Source: CAD feature listing. Evaluate the final solid. Frame: model axes, mm. A direction names the side the tool comes from. Give positions to 0.01 mm unless a question says otherwise; leave off trailing zeros. Order: outer loops, then holes, each group sorted by start corner. A loop starts at its lowest first (then second) coordinate and runs counter-clockwise, first axis right, second up.
from build123d import *

# Parameters (mm, degrees)
SKETCH_W        = 108
SKETCH_H        = 38
PAD_DEPTH       = 3
SKETCH002_W     = 3
SKETCH002_H     = 38
POCKET_DEPTH    = 1.5
SKETCH003_W     = 3
SKETCH003_H     = 38
POCKET001_DEPTH = 1.5
SKETCH004_W     = 102
SKETCH004_H     = 1.5
POCKET002_DEPTH = 1.5
SKETCH005_W     = 102
SKETCH005_H     = 1.5
POCKET003_DEPTH = 1.5
SKETCH006_W     = 5
SKETCH006_H     = 5
POCKET004_DEPTH = 3


with BuildPart() as part:
    # Sketch → Pad (new body)
    with BuildSketch(Plane.XY):
        with Locations((54, -19)):
            Rectangle(SKETCH_W, SKETCH_H)
    extrude(amount=PAD_DEPTH)

    # Sketch002 (on Face6 of Pad) → Pocket (cut)
    with BuildSketch(Plane.XY.offset(3)):
        with Locations((1.5, -19)):
            Rectangle(SKETCH002_W, SKETCH002_H)
    extrude(amount=-POCKET_DEPTH, mode=Mode.SUBTRACT)

    # Sketch003 (on Face4 of Pocket) → Pocket001 (cut)
    with BuildSketch(Plane.XY.offset(3)):
        with Locations((106.5, -19)):
            Rectangle(SKETCH003_W, SKETCH003_H)
    extrude(amount=-POCKET001_DEPTH, mode=Mode.SUBTRACT)

    # Sketch004 (on Face6 of Pocket001) → Pocket002 (cut)
    with BuildSketch(Plane.XY.offset(3)):
        with Locations((54, -0.75)):
            Rectangle(SKETCH004_W, SKETCH004_H)
    extrude(amount=-POCKET002_DEPTH, mode=Mode.SUBTRACT)

    # Sketch005 (on Face12 of Pocket002) → Pocket003 (cut)
    with BuildSketch(Plane.XY.offset(3)):
        with Locations((54, -37.25)):
            Rectangle(SKETCH005_W, SKETCH005_H)
    extrude(amount=-POCKET003_DEPTH, mode=Mode.SUBTRACT)

    # Sketch006 (on Face13 of Pocket003) → Pocket004 (cut)
    with BuildSketch(Plane.XY.offset(3)):
        with Locations((6.75, -16.25)):
            Rectangle(SKETCH006_W, SKETCH006_H)
    extrude(amount=-POCKET004_DEPTH, mode=Mode.SUBTRACT)


solid = part.part
1) Section query A-A on y = -17. Output: boundary loops of the cut face in (x, z), and give its area (3 significant figures).
Checks:
outline: (0, 0) - (4.25, 0) - (4.25, 3) - (3, 3) - (3, 1.5) - (0, 1.5) - close; (9.25, 0) - (108, 0) - (108, 1.5) - (105, 1.5) - (105, 3) - (9.25, 3) - close
area: 300 mm2
2) Ray query, L1, parallel to X at y = -22.5, z = 2.05; L2, parallel to X at y = -14, z = 2.9; L3, parallel to Y at x = 88, z = 2.55. Return the intervals inside material, ascending.
Checks:
L1: x = 3 to 105
L2: x = 3 to 4.25, 9.25 to 105
L3: y = -36.5 to -1.5
3) Reachability of faces 1 (the face through (9.25, -16, 2)), 2 (the face through (53, -19, 0)) from +Z, -Z, +X, -X, +Y, -Y: full face, straight path, thin tool, end or side. Return the list, or none.
Checks:
face 1: +Z, -Z
face 2: -Z, +X, -X, +Y, -Y
4) Pull-direction query (Y, two-part tool) for faces 3 (the face through (4.25, -16, 2)), 4 (the face through (50, -37, 1.5)); classes: +Y half, -Y half, draft (parallel to the pull), parting line (faces both ways), or undercut.
Checks:
face 3: undercut
face 4: draft
5) Section query D-D on y = -5. Output: boundary loops of the cut face in (x, z), and give its area (3 significant figures).
Checks:
outline: (0, 0) - (108, 0) - (108, 1.5) - (105, 1.5) - (105, 3) - (3, 3) - (3, 1.5) - (0, 1.5) - close
area: 315 mm2
6) Section query C-C on x = 44. Output: boundary loops of the cut face in (y, z), and give its area (4 significant figures).
Checks:
outline: (-38, 0) - (0, 0) - (0, 1.5) - (-1.5, 1.5) - (-1.5, 3) - (-36.5, 3) - (-36.5, 1.5) - (-38, 1.5) - close
area: 109.5 mm2
7) Section query B-B on z = 2.15. Output: boundary loops of the cut face in (x, y).
Checks:
outline: (3, -36.5) - (105, -36.5) - (105, -1.5) - (3, -1.5) - close; hole (4.25, -18.75) - (9.25, -18.75) - (9.25, -13.75) - (4.25, -13.75) - close
8) First-contact query: pin 1 Ø1.2 at (x, z) = (70, 2) entering from +Y; pin 2 Ø1.6 at (y, z) = (-12, 2.5) entering from -X; pin 3 Ø0.8 at (y, z) = (-14, 2.5) entering from +X. Flat tips, straight axial feed; report the tip coordinate or a pass-through.
Checks:
pin 1: stops at y = 0
pin 2: stops at x = 3
pin 3: stops at x = 105
